For this review, take the finished solid that the model builds, in its own axes (mm). Face numbers are marked on the shaded views. A direction names the side the tool comes from. Coordinates: 2 decimals unless noted, no trailing zeros. Write each loop counter-clockwise with the first axis right and the second up, starting at its lowest first coordinate (ties: lowest second). Pieces come first, ordered by that corner, then holes.
1) For the marked faces 4 and 5, list the 3-axis set-ups (+Z, -Z, +X, -X, +Y, -Y) from which the entire face can be reached by the end or side of a thin tool; tool diameter is ignored.
2) Mouldability with a two-part tool opening along X and no side actions: class the marked faces 1, 2 and 3 as pulls with the +X half, pulls with the -X half, needs draft (parallel to the pull), parting line crosses it, or undercut.
3) We need section D-D on x = 4. Write out the cut boundary in (y, z).
4) To check wall thickness, follow line 1 along X through (y, z) = (-0.5, 2.5); line 2 along Z through (x, y) = (4, -2.5); line 3 along Y through (x, z) = (1.5, 4.5). State the ranges of each line that lie inside material, in increasing order.
5) Insertion check: P1, Ø5, axis at x = 4, y = -1.5, coming from the +Z side; P2, Ø4, axis at x = -10.63, z = 22, coming from the -Y side; P3, Ø2, axis at x = 10.5, y = 0, coming from the -Z side; P4, Ø3.5, axis at y = 4.5, z = 7.5, coming from the -X side. Each pin has a flat end and moves straight along its axis. Give the tip position at first contact, or say it passes through.
6) We need section C-C on z = 22. Write out the cut boundary in (x, y), then the cut area to 3 significant figures.
7) We need section B-B on x = 11.5. Write out the cut boundary in (y, z), then the cut area to 3 significant figures.
8) We need section A-A on y = 0. Write out the cut boundary in (x, z), then the cut area to 3 significant figures.
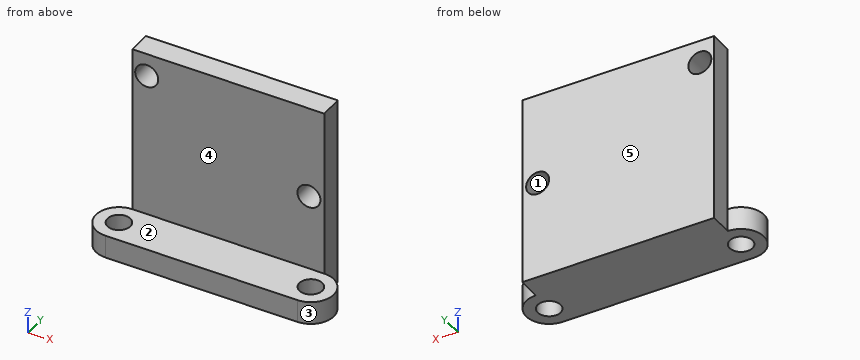
from build123d import *

# Parameters (mm, degrees)
SKETCH_1_R          = 1.5
EXTRUDE_1_DEPTH     = 3
EXTRUDE_START       = -3
SKETCH_2_W          = 25
SKETCH_2_H          = 3
EXTRUDE_2_DEPTH     = 25
SKETCH_8_R          = 1.5
CUT_EXTRUDE_1_DEPTH = 31.020826105


with BuildPart() as part:
    # 草图1 → 凸台-拉伸1 (new body)
    with BuildSketch(Plane.XY):
        with BuildLine():
            Line((12.5, 3), (-12.5, 3))
            ThreePointArc((-12.5, 3), (-15.5, 0), (-12.5, -3))
            Line((-12.5, -3), (12.5, -3))
            ThreePointArc((12.5, -3), (15.5, 0), (12.5, 3))
        make_face()
        with Locations((-12.5, 0)):
            Circle(SKETCH_1_R, mode=Mode.SUBTRACT)
        with Locations((12.5, 0)):
            Circle(SKETCH_1_R, mode=Mode.SUBTRACT)
    extrude(amount=EXTRUDE_1_DEPTH)

    # 草图2 → 凸台-拉伸2 (add)
    with BuildSketch(Plane.XY.offset(3).offset(EXTRUDE_START)):
        with Locations((0, 4.5)):
            Rectangle(SKETCH_2_W, SKETCH_2_H)
    extrude(amount=EXTRUDE_2_DEPTH)

    # 草图8 → 切除-拉伸1 (cut, through all)
    with BuildSketch(Plane.XZ.offset(-3)):
        with Locations(Location((-10.629379797, 22, 0), (0, 0, 270))):
            Circle(SKETCH_8_R)
        with Locations(Location((10.50249981, 12.920150648, 0), (0, 0, 270))):
            Circle(SKETCH_8_R)
    extrude(amount=-CUT_EXTRUDE_1_DEPTH, mode=Mode.SUBTRACT)


solid = part.part
Result:
1. face 4: +Z, +X, -X, -Y
1. face 5: +Z, -Z, +X, -X, +Y
2. face 1: undercut
2. face 2: needs draft
2. face 3: pulls with the +X half
3. outline: (-3, 0) - (6, 0) - (6, 25) - (3, 25) - (3, 3) - (-3, 3) - close
4. line 1: x = -15.46 to -13.91, -11.09 to 11.09, 13.91 to 15.46
4. line 2: z = 0 to 3
4. line 3: y = 3 to 6
5. P1: stops at z = 3
5. P2: stops at y = 3
5. P3: stops at z = 0
5. P4: stops at x = -12.5
6. outline: (-12.5, 3) - (-12.13, 3) - (-12.13, 6) - (-12.5, 6) - close; (-9.13, 3) - (12.5, 3) - (12.5, 6) - (-9.13, 6) - close
6. area: 66.0 mm2
7. outline: (-3, 0) - (-1.12, 0) - (-1.12, 3) - (-3, 3) - close; (1.12, 0) - (6, 0) - (6, 11.8) - (3, 11.8) - (3, 3) - (1.12, 3) - close; (3, 14.04) - (6, 14.04) - (6, 25) - (3, 25) - close
7. area: 79.6 mm2
8. outline: (-15.5, 0) - (-14, 0) - (-14, 3) - (-15.5, 3) - close; (-11, 0) - (11, 0) - (11, 3) - (-11, 3) - close; (14, 0) - (15.5, 0) - (15.5, 3) - (14, 3) - close
8. area: 75.0 mm2
